from build123d import *

# Parameters (mm, degrees)
SKETCH_R           = 48.380289
PAD_DEPTH          = 10
POCKET_DEPTH       = 3
POCKET001_DEPTH    = 2.5
POLARPATTERN_COUNT = 2


with BuildPart() as part:
    # Sketch → Pad (new body)
    with BuildSketch(Plane.XY):
        Circle(SKETCH_R)
    extrude(amount=PAD_DEPTH)

    # Sketch001 (on Face3 of Pad) → Pocket (cut)
    with BuildSketch(Plane.XY.offset(10)):
        with BuildLine():
            ThreePointArc((2.048306, 31.433333), (-2.49861, 30.083359), (1.948219, 28.433333))
            ThreePointArc((5.438052, 27.976376), (3.700196, 28.258778), (1.948219, 28.433333))
            ThreePointArc((5.438052, 27.976376), (7.19671, 29.162599), (6.010484, 30.921256))
            ThreePointArc((6.010484, 30.921256), (4.037521, 31.240173), (2.048306, 31.433333))
        make_face()
    pocket = extrude(amount=-POCKET_DEPTH, mode=Mode.SUBTRACT)

    # Sketch002 (on Face3 of Pocket) → Pocket001 (cut)
    with BuildSketch(Plane.XY.offset(9)):
        with BuildLine():
            ThreePointArc((0.239614, 32.48849), (-2.48849, 30.239614), (-0.239614, 27.51151))
            Line((-0.239614, 27.51151), (5.484655, 26.960325))
            ThreePointArc((5.484655, 26.960325), (8.21276, 29.209201), (5.963884, 31.937306))
            Line((5.963884, 31.937306), (0.239614, 32.48849))
        make_face()
    pocket001 = extrude(amount=-POCKET001_DEPTH, mode=Mode.SUBTRACT)

    # PolarPattern: Pocket, Pocket001 ×2 about axis
    polarpattern_axis = Axis((0, 0, 10), (0, 0, 1))
    for i in range(1, POLARPATTERN_COUNT):
        add(pocket.rotate(polarpattern_axis, i * 360 / POLARPATTERN_COUNT), mode=Mode.SUBTRACT)
        add(pocket001.rotate(polarpattern_axis, i * 360 / POLARPATTERN_COUNT), mode=Mode.SUBTRACT)


solid = part.part
Can you work these out from the model? Positions are in its coordinate system, mm. A direction names the side the tool comes from. Give positions to 0.01 mm unless a question says otherwise; leave off trailing zeros. Loops run counter-clockwise (first coordinate to the right, second up) from the corner with the lowest first, then second, coordinate; pieces in that order, holes last. Notation, with made-up numbers: (39, 50) - (78, 50) arc R26 ccw to (78, 81) - close; hole circle Ø2 at (-37, -0.75). An arc over 180 degrees is marked (long way). Answer as a JSON object with one key per item and string values.
Q1. Imagine slicing it at A-A on z = 2.25. Write out the boundary of the cut face in (x, y).
Geometry says:
{"outline": "circle Ø96.76 at (0, 0)"}
Q2. Which directions (+Z, -Z, +X, -X, +Y, -Y) give clear straight access to the entire face, cutting with the end or side of a thin tool? Please do faces 4 (the cylindrical face through (2.494, -30.171, 8.854)), 5 (the flat face through (-1, 1, 0)), 6 (the flat face through (-3, -30, 6.5)).
Geometry says:
{"face 4": "+Z", "face 5": "-Z, +X, -X, +Y, -Y", "face 6": "none"}
Q3. If I drill on L1, parallel to Y at x = 0, z = 7.85; L2, parallel to X at y = 30, z = 9.15; L3, parallel to X at y = -30, z = 8.85, over which ranges is the centre line in solid material (lowest first)?
Geometry says:
{"L1": "-48.38 to -32.5, -27.49 to 27.49, 32.5 to 48.38", "L2": "-37.96 to -2.5, 7.12 to 37.96", "L3": "-37.96 to -8.16, 2.5 to 37.96"}
Q4. Imagine slicing it at B-B on x = 33. Write out the boundary of the cut face in (y, z).
Geometry says:
{"outline": "(-35.38, 0) - (35.38, 0) - (35.38, 10) - (-35.38, 10) - close"}
Q5. If we mould it in two halves opening along Y, with no side actions, what happens to faces 1 (the cylindrical face through (46.146, 14.532, 4.93)), 2 (the flat face through (-1, 1, 10)), 3 (the cylindrical face through (-2.494, 30.171, 8.854))? For each: pulls with the +Y half, pulls with the -Y half, needs draft (parallel to the pull), parting line crosses it, or undercut.
Geometry says:
{"face 1": "parting line crosses it", "face 2": "needs draft", "face 3": "undercut"}
Q6. Imagine slicing it at C-C on y = 42. Write out the boundary of the cut face in (x, z).
Geometry says:
{"outline": "(-24.01, 0) - (24.01, 0) - (24.01, 10) - (-24.01, 10) - close"}
Q7. Will these pins go through, and if not, where does the flat tip stop? P1, Ø5, axis at x = -11.5, z = 8, coming from the -Y side; P2, Ø3, axis at x = 33.5, z = 7.5, coming from the -Y side; P3, Ø6, axis at y = 36, z = 1.5, coming from the -X side.
Geometry says:
{"P1": "y = -47.54", "P2": "y = -36.29", "P3": "x = -35.38"}
